Can you work these out from the drawing? Everything is in mm from the part's minimum corner. Round coordinates to 2 decimals unless told otherwise and drop trailing zeros. Loops run counter-clockwise (first coordinate to the right, second up) from the corner with the lowest first, then second, coordinate; pieces in that order, holes last. Notation, with made-up numbers: (20.25, 2) - (34.25, 2) arc R9 ccw to (34.25, 17) - close; hole circle Ø5 at (-12.5, 26.5). An arc over 180 degrees is marked (long way). Answer as a JSON object with one key per item and string values. Group by question number.
1) I want a section at C-C, the plane y = 18. Please give me the cut outline in (x, z), then the cut area to 3 significant figures.
2) Will these pins go through, and if not, where does the flat tip stop? P1, Ø1.3, axis at x = 42.5, y = 25.5, coming from the -Z side; P2, Ø10, axis at x = 38, y = 12, coming from the -Z side; P3, Ø1.5, axis at y = 31, z = 33.5, coming from the -X side.
3) If we mould it in two halves opening along X, with no side actions, what happens to the marked faces 1 and 2? For each: pulls with the +X half, pulls with the -X half, needs draft (parallel to the pull), parting line crosses it, or undercut.
4) I want a section at A-A, the plane x = 23. Please give me the cut outline in (y, z).
5) I want a section at B-B, the plane z = 23. Please give me the cut outline in (x, y).
6) If I drill on line 1 along Z through (x, y) = (23, 16); line 2 along X through (y, z) = (8, 23.5); line 3 along Z through (x, y) = (4.5, 6), over which ranges is the centre line in solid material (lowest first)? Write a range as [from, to].
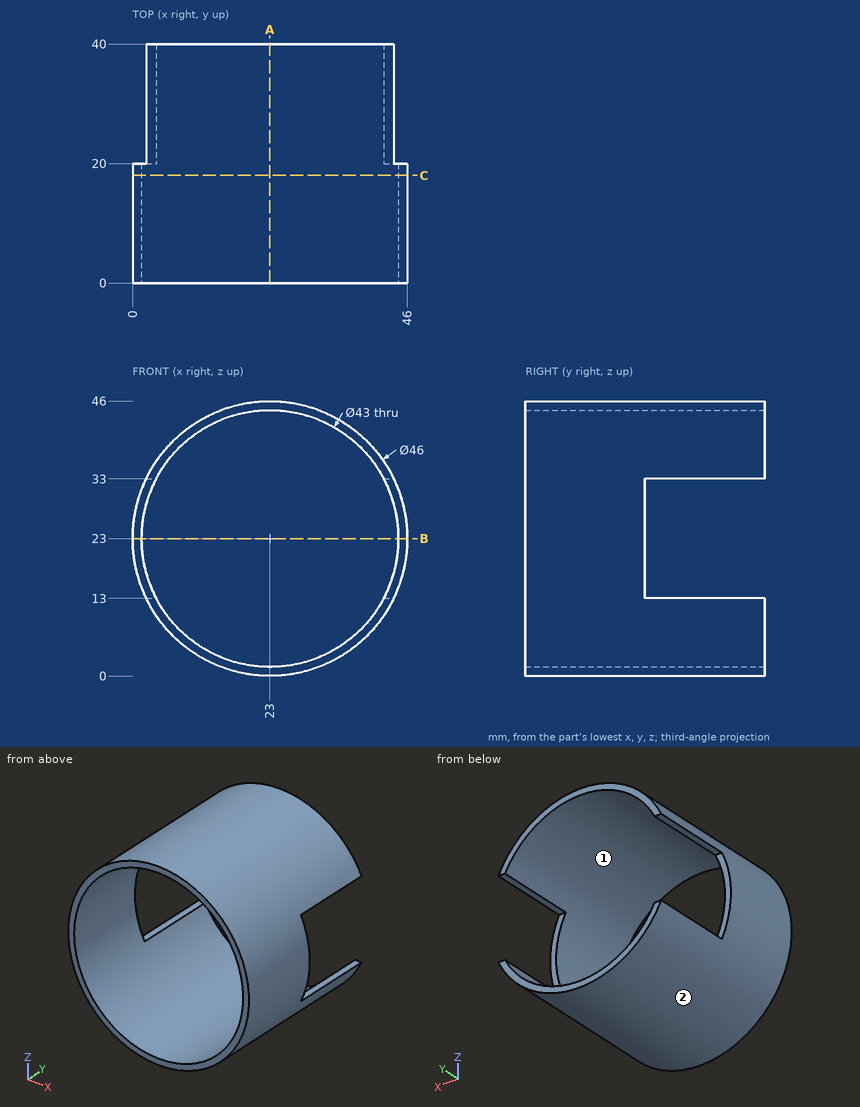
Outcome:
{
 "1": {"outline": "circle Ø46 at (23, 23); hole circle Ø43 at (23, 23)", "area": "210 mm^2"},
 "2": {"P1": "z = 9.82", "P2": "z = 2.29", "P3": "x = 2.29"},
 "3": {"face 1": "undercut", "face 2": "parting line crosses it"},
 "4": {"outline": "(0, 0) - (40, 0) - (40, 1.5) - (0, 1.5) - close; (0, 44.5) - (40, 44.5) - (40, 46) - (0, 46) - close"},
 "5": {"outline": "(0, 0) - (1.5, 0) - (1.5, 20) - (0, 20) - close; (44.5, 0) - (46, 0) - (46, 20) - (44.5, 20) - close"},
 "6": {"line 1": "[0, 1.5], [44.5, 46]", "line 2": "[0.01, 1.51], [44.49, 45.99]", "line 3": "[9.33, 12.05], [33.95, 36.67]"}
}
